For this review, take the finished solid that the model builds, in its own axes (mm). Coordinates: 2 decimals unless noted, no trailing zeros. Write each loop counter-clockwise with the first axis right and the second up, starting at its lowest first coordinate (ties: lowest second). Pieces come first, ordered by that corner, then holes. Notation, with made-up numbers: M 33,24.25 L 69,24.25 A3 cw 69,28.25 Z; hole C 65,-9.75 d5. An arc over 180 degrees is marked long. One line per question, with ' | ' between items.
Autodesk Inventor part; units mm, degrees
ref_plane "YZ Plane" through (0, 0, 0) normal (1, 0, 0) x (0, 1, 0)
ref_plane "XZ Plane" through (0, 0, 0) normal (0, 1, 0) x (-1, 0, 0)
ref_plane "XY Plane" through (0, 0, 0) normal (0, 0, 1) x (1, 0, 0)
sketch "Sketch1" plane through (0, 0, 0) normal (0, 1, 0) x (-1, 0, 0)
  line L0 (0, 0) -> (317, 0)
  line L1 (317, 0) -> (317, 25)
  line L2 (317, 25) -> (0, 25)
  line L3 (0, 25) -> (0, 0)
  dimension "d0" = 317
  dimension "d1" = 25
extrude "Extrusion1" add sketch "Sketch1" along normal blind 100
fillet "Face Fillet1" radius 2 1 edges at (-317, 50, 0)
sketch "Sketch5" plane through (0, 0, 0) normal (0, 1, 0) x (-1, 0, 0)
  circle A0 centre (15.133, 12.0626) radius 7.2608
  circle A1 centre (76.981, 12.0626) radius 7.5
  circle A2 centre (160.761, 12.0626) radius 7.5
  circle A3 centre (268.666, 12.0626) radius 10.0887
  point P0 (0, 0)
  dimension "d16" = 15
  dimension "d17" = 15
extrude "Extrusion4" cut sketch "Sketch5" along normal blind 100
sketch "Sketch6" plane through (-317, 0, 25) normal (-1, 0, 0) x (0, 0, 1)
  point P0 (-25, 0)
properties part number "BASE"
1. Clearance check with a flat-ended pin moving along its axis: P1, Ø8.5, axis at x = -15.13, z = 12.06, coming from the -Y side. State where the tip first meets the part, or that it passes through.
Computed values:
P1: passes through
2. Take a section at A-A on z = 15.5. State the section outline as (x, y) points, plus the area to 3 significant figures.
Computed values:
outline: M -317,0 L -278.15,0 L -278.15,100 L -317,100 Z; M -259.18,0 L -167.43,0 L -167.43,100 L -259.18,100 Z; M -154.1,0 L -83.65,0 L -83.65,100 L -154.1,100 Z; M -70.32,0 L -21.53,0 L -21.53,100 L -70.32,100 Z; M -8.74,0 L 0,0 L 0,100 L -8.74,100 Z | area: 25,900 mm2
3. Draft analysis for pull direction X (two halves, no side actions). For faces 1 (the flat face through (0, 49, 13)), 2 (the cylindrical face through (-69.49, 49.3, 11.73)), 3 (the flat face through (-161, 49, 25)), state which applies: pulls with the +X half, pulls with the -X half, needs draft (parallel to the pull), parting line crosses it, or undercut.
Computed values:
face 1: pulls with the +X half | face 2: undercut | face 3: needs draft
4. Take a section at C-C on y = 53.5. State the section outline as (x, z) points.
Computed values:
outline: M -317,2 A2 ccw -315,0 L 0,0 L 0,25 L -317,25 Z; hole C -268.67,12.06 d20.18; hole C -160.76,12.06 d15; hole C -76.98,12.06 d15; hole C -15.13,12.06 d14.52
5. For line 1 along X through (y, z) = (26, 12.75); line 2 along X through (y, z) = (20, 12.25); line 3 along Z through (x, y) = (-76.5, 18), list the stretches that pass through material, from the lowest coordinate up.
Computed values:
line 1: x = -317 to -278.73, -258.6 to -168.23, -153.29 to -84.45, -69.51 to -22.36, -7.9 to 0 | line 2: x = -317 to -278.75, -258.58 to -168.26, -153.26 to -84.48, -69.48 to -22.39, -7.87 to 0 | line 3: z = 0 to 4.58, 19.55 to 25
6. Take a section at B-B on x = -77. State the section outline as (y, z) points.
Computed values:
outline: M 0,0 L 100,0 L 100,4.56 L 0,4.56 Z; M 0,19.56 L 100,19.56 L 100,25 L 0,25 Z
